Drawing for the job (mm, zero at the part's lowest x, y, z). Round coordinates to 2 decimals unless told otherwise and drop trailing zeros. Write each loop counter-clockwise with the first axis right and the second up, starting at its lowest first coordinate (ties: lowest second). Pieces come first, ordered by that corner, then holes. Notation, with made-up numbers: M 21.5,-30 L 49.5,-30 A13 ccw 49.5,-11 Z; hole C 77,74.25 d9. An arc over 180 degrees is marked long. Use a Markdown table: item, result.
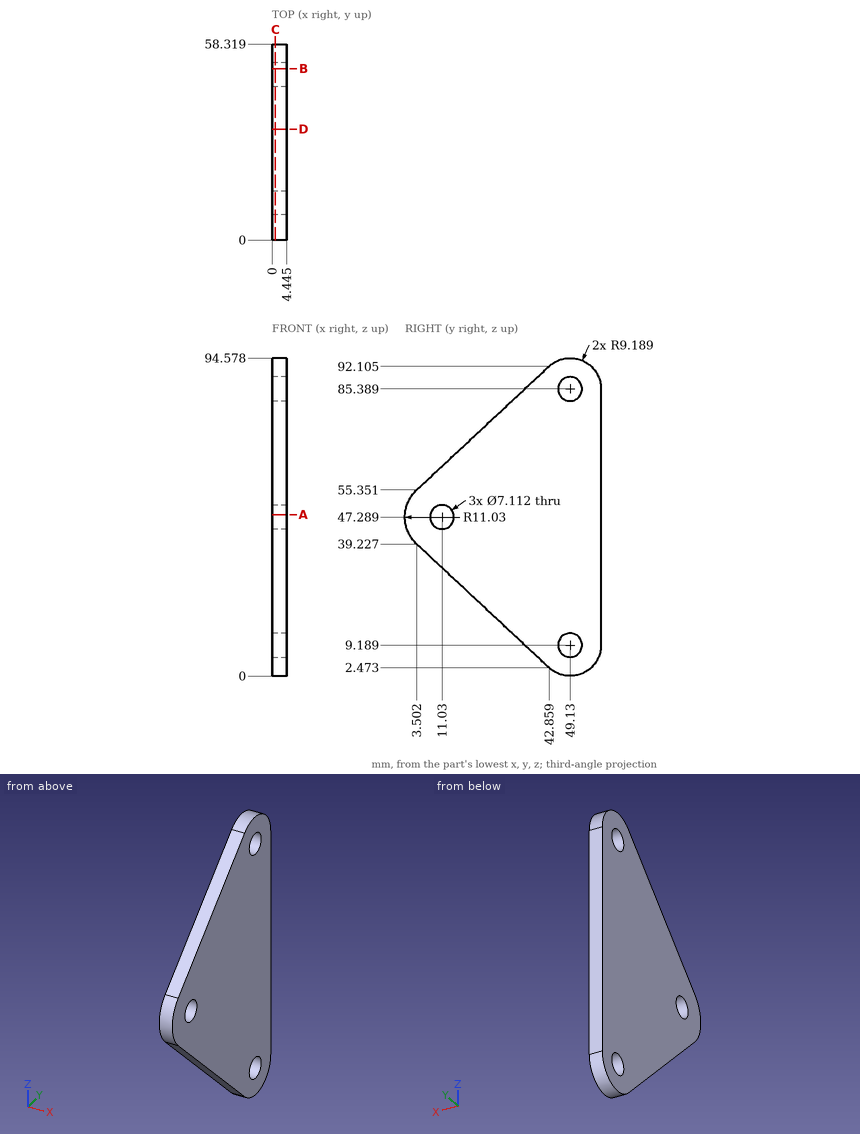
Q1. Cut at A-A on z = 48. Give the cut face in (x, y) (1 decimal).
Response values:
| item | result |
|---|---|
| outline | M 0,0 L 4.4,0 L 4.4,7.5 L 0,7.5 Z; M 0,14.5 L 4.4,14.5 L 4.4,58.3 L 0,58.3 Z |
Q2. Cut at D-D on y = 33. Give the cut face in (x, z) (1 decimal).
Response values:
| item | result |
|---|---|
| outline | M 0,11.7 L 4.4,11.7 L 4.4,82.9 L 0,82.9 Z |
Q3. Drill centre lines: L1, parallel to Z at x = 3.7, y = 50.5 (1 decimal); L2, parallel to Y at x = 1.55, z = 59; L3, parallel to Y at x = 1.6, z = 71.5 (1 decimal). Where is each one in solid material? Low to high.
Response values:
| item | result |
|---|---|
| L1 | z = 0.1 to 5.9, 12.5 to 82.1, 88.7 to 94.5 |
| L2 | y = 7.41 to 58.32 |
| L3 | y = 20.8 to 58.3 |
Q4. Cut at C-C on x = 1. Count the separate pieces of the cut face and the enclosed holes in it, and give its area (3 significant figures).
Response values:
| item | result |
|---|---|
| separate pieces | 1 |
| enclosed holes | 3 |
| area | 3,420 mm2 |
Q5. Cut at B-B on y = 51. Give the cut face in (x, z) (1 decimal), and give its area (3 significant figures).
Response values:
| item | result |
|---|---|
| outline | M 0,0.2 L 4.4,0.2 L 4.4,6.2 L 0,6.2 Z; M 0,12.2 L 4.4,12.2 L 4.4,82.4 L 0,82.4 Z; M 0,88.4 L 4.4,88.4 L 4.4,94.4 L 0,94.4 Z |
| area | 365 mm2 |
Q6. Drop flat-ended pins along their axis: P1, Ø6.5, axis at y = 49.13, z = 85.39, coming from the -X side; P2, Ø1, axis at x = 0.5, y = 27, coming from the -Z side (1 decimal); P3, Ø1, axis at x = 1.5, y = 24.5, coming from the -Z side. Give the stop position or say it passes through.
Response values:
| item | result |
|---|---|
| P1 | passes through |
| P2 | stops at z = 16.8 |
| P3 | stops at z = 19.15 |
